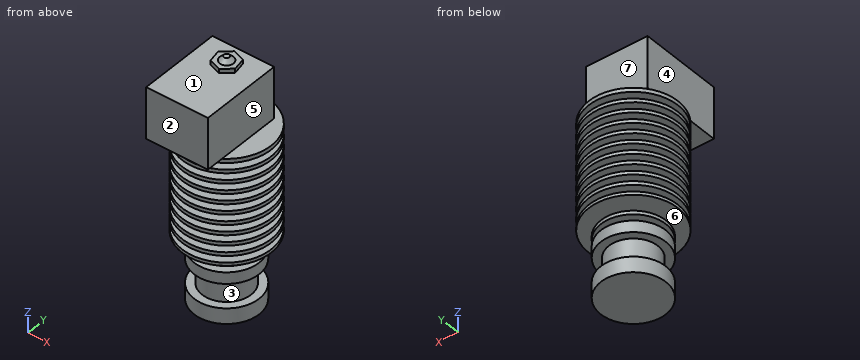
from build123d import *

# Parameters (mm, degrees)
SKETCH1_R           = 10.845
BOSS_EXTRUDE1_DEPTH = 25.9
SKETCH2_W           = 5.345
SKETCH2_H           = 1.6
LPATTERN1_COUNT     = 10
LPATTERN1_PITCH     = 2.5
SKETCH3_R           = 7.9
BOSS_EXTRUDE2_DEPTH = 16.4
SKETCH4_W           = 1.95
SKETCH4_H           = 5.92
SKETCH4_W_2         = 2.9
SKETCH4_H_2         = 1.5
SKETCH5_R           = 2
BOSS_EXTRUDE3_DEPTH = 1.8
SKETCH6_W           = 15
SKETCH6_H           = 20
BOSS_EXTRUDE4_DEPTH = 12.5
BOSS_EXTRUDE5_DEPTH = 1
SKETCH8_R           = 1.65934661
BOSS_EXTRUDE6_DEPTH = 1
BOSS_EXTRUDE6_TAPER = 45


with BuildPart() as part:
    # Sketch1 → Boss-Extrude1 (new body)
    with BuildSketch(Plane.XY):
        with Locations(Location((0, 0, 0), (0, 0, 180))):
            Circle(SKETCH1_R)
    extrude(amount=BOSS_EXTRUDE1_DEPTH)

    # Sketch2 → Cut-Revolve1 (revolve, cut)
    with BuildSketch(Plane(origin=(0, 0, 0), x_dir=(1, 0, 0), z_dir=(0, 1, 0))):
        with Locations((-8.1725, -1.6)):
            Rectangle(SKETCH2_W, SKETCH2_H)
    cut_revolve1 = revolve(axis=Axis((0, 0, 0), (0, 0, 1)), mode=Mode.SUBTRACT)

    # LPattern1: Cut-Revolve1 ×10
    with Locations(*[(0, 0, i * LPATTERN1_PITCH) for i in range(1, LPATTERN1_COUNT)]):
        add(cut_revolve1, mode=Mode.SUBTRACT)

    # Sketch3 → Boss-Extrude2 (add)
    with BuildSketch(Plane(origin=(0, 0, 0), x_dir=(-1, 0, 0), z_dir=(0, 0, -1))):
        with Locations(Location((0, 0, 0), (0, 0, 180))):
            Circle(SKETCH3_R)
    extrude(amount=BOSS_EXTRUDE2_DEPTH)

    # Sketch4 → Cut-Revolve2 (revolve, cut)
    with BuildSketch(Plane(origin=(0, 0, 0), x_dir=(1, 0, 0), z_dir=(0, 1, 0)), mode=Mode.PRIVATE) as cut_revolve2_sk:
        with Locations((-6.925, 9.66)):
            Rectangle(SKETCH4_W, SKETCH4_H)
        with Locations((-6.45, 3.15)):
            Rectangle(SKETCH4_W_2, SKETCH4_H_2)
        with Locations((-6.45, 0.75)):
            Rectangle(SKETCH4_W_2, SKETCH4_H_2)
    revolve(cut_revolve2_sk.sketch.rotate(Axis((0, 0, 0), (0, 0, -1)), 180), axis=Axis((0, 0, 0), (0, 0, -1)), mode=Mode.SUBTRACT)

    # Sketch5 → Boss-Extrude3 (add)
    with BuildSketch(Plane.XY.offset(25.9)):
        Circle(SKETCH5_R)
    extrude(amount=BOSS_EXTRUDE3_DEPTH)

    # Sketch6 → Boss-Extrude4 (add)
    with BuildSketch(Plane.XY.offset(27.7)):
        with Locations((0, -5)):
            Rectangle(SKETCH6_W, SKETCH6_H)
    extrude(amount=BOSS_EXTRUDE4_DEPTH)

    # Sketch7 → Boss-Extrude5 (add)
    with BuildSketch(Plane.XY.offset(40.2)):
        Polygon((2.891396573, -1.018451956), (2.327703553, 1.994796907), (-0.56369302, 3.013248863), (-2.891396573, 1.018451956), (-2.327703553, -1.994796907), (0.56369302, -3.013248863), align=None)
    extrude(amount=BOSS_EXTRUDE5_DEPTH)

    # Sketch8 → Boss-Extrude6 (add)
    with BuildSketch(Plane.XY.offset(41.2)):
        Circle(SKETCH8_R)
    extrude(amount=BOSS_EXTRUDE6_DEPTH, taper=BOSS_EXTRUDE6_TAPER)


solid = part.part
The listing builds one solid part. Answer for the finished solid, in the listing's coordinates (mm). Face numbers are marked on the shaded views. A direction names the side the tool comes from. Give positions to 0.01 mm unless a question says otherwise; leave off trailing zeros. Write each loop counter-clockwise with the first axis right and the second up, starting at its lowest first coordinate (ties: lowest second). Pieces come first, ordered by that corner, then holes. Notation, with made-up numbers: (45.5, -39) -> (56.5, -39) arc R12 cw to (56.5, -18) -> close; hole circle Ø1 at (-10, -1.5). An arc over 180 degrees is marked (long way). One line per question, with ' | ' between items. Start each with the question number.
1. Section C-C (z = 29.5) is taken. Determine the outline of the cut face in (x, y), plus the area to 3 significant figures.
2. For a pull along Z with two mould halves and no side action, classify the marked faces 1, 2 and 3 as pulls with the +Z half, pulls with the -Z half, needs draft (parallel to the pull), parting line crosses it, or undercut.
3. For the marked faces 4, 5, 6 and 7, determine the directions among +Z, -Z, +X, -X, +Y, -Y from which every point of the face is accessible in a straight line to the end or side of a thin tool.
4. Given pin 1 Ø1.5 at (x, y) = (4.5, -3) entering from +Z; pin 2 Ø1 at (x, y) = (-5.5, 6.5) entering from +Z; pin 3 Ø3 at (x, z) = (-6, -5) entering from +Y; pin 4 Ø11 at (x, y) = (3.5, -3) entering from +Z, each flat-ended and moving along its own axis, determine where each tip first touches the part or whether it passes through.
5. Find the intervals of material crossed by probe 1 along Z at (x, y) = (0, 3.25); probe 2 along Z at (x, y) = (1.75, 2); probe 3 along X at (y, z) = (-7.25, 36.5), in increasing order.
6. Section A-A (z = 9) is taken. Determine the outline of the cut face in (x, y), plus the area to 3 significant figures.
7. Section B-B (y = -10.25) is taken. State how many separate pieces and enclosed holes the cut face has, plus the area to 3 significant figures.
Response values:
1) outline: (-7.5, -15) -> (7.5, -15) -> (7.5, 5) -> (-7.5, 5) -> close | area: 300 mm2
2) face 1: pulls with the +Z half | face 2: needs draft | face 3: undercut
3) face 4: +Z, -X, +Y, -Y | face 5: +Z, +X, +Y, -Y | face 6: none | face 7: +Z, +X, -X, +Y
4) pin 1: z = 40.2 | pin 2: z = 25.9 | pin 3: y = 6.49 | pin 4: z = 42.2
5) probe 1: -16.4 to 25.9, 27.7 to 40.2 | probe 2: -16.4 to 25.9, 27.7 to 41.2 | probe 3: -7.5 to 7.5
6) outline: circle Ø11 at (0, 0) | area: 95.0 mm2
7) separate pieces: 12 | enclosed holes: 0 | area: 258 mm2
